Drawing for the job (mm, zero at the part's lowest x, y, z). A direction names the side the tool comes from. Coordinates: 2 decimals unless noted, no trailing zeros. Write each loop counter-clockwise with the first axis right and the second up, starting at its lowest first coordinate (ties: lowest second). Pieces come first, ordered by that corner, then holes. Notation, with made-up numbers: (33, 78.5) -> (71, 78.5) arc R29 ccw to (71, 105.5) -> close; hole circle Ø1 at (-29.5, 68). An arc over 180 degrees is marked (long way). Answer as CSV lines item,"result".
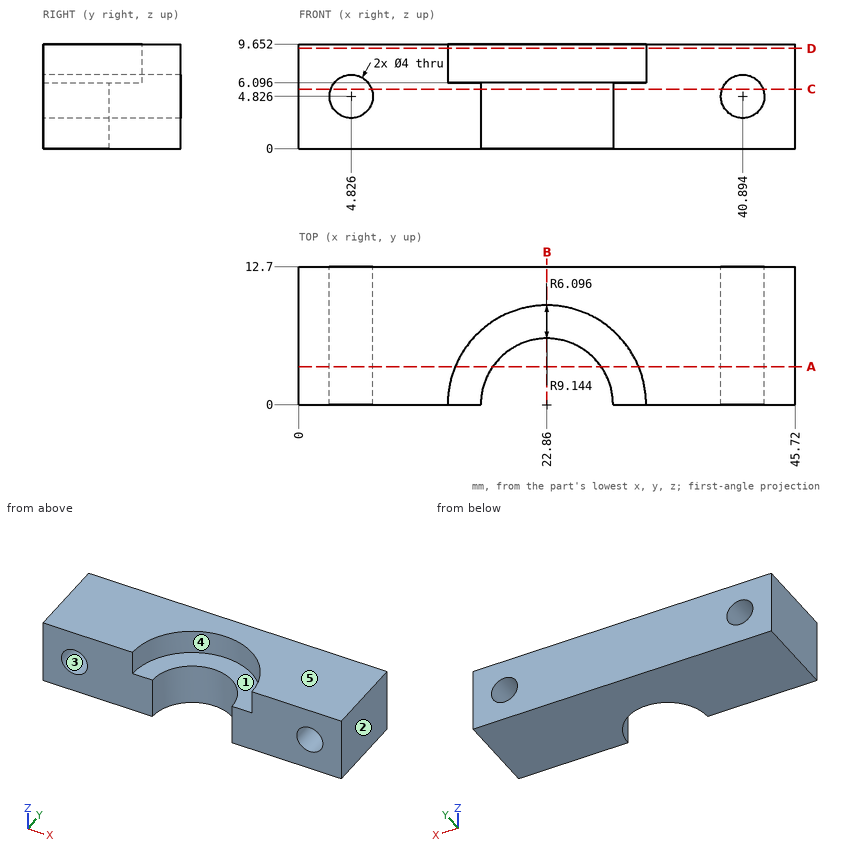
Item 1: Two-plate mould, pull along Z, no slides. Class the marked faces 3, 4 and 5: pulls with the +Z half, pulls with the -Z half, needs draft (parallel to the pull), parting line crosses it, or undercut.
Answer below:
face 3,"undercut"
face 4,"needs draft"
face 5,"pulls with the +Z half"
Item 2: 3-axis set-ups, long thin cutter, end or side, ignore diameter. For the marked faces 1 and 2: which of +Z, -Z, +X, -X, +Y, -Y reach the whole face in a straight line?
Answer below:
face 1,"+Z, -Y"
face 2,"+Z, -Z, +X, +Y, -Y"
Item 3: Wall check: line 1 (X direction, y = 8.5, z = 5); line 2 (X direction, y = 5.5, z = 6.5); line 3 (X direction, y = 3.75, z = 4.5). Give the ranges that are in metal, low to high. Write a range as from..to.
Answer below:
line 1,"x = 0..2.83, 6.82..38.9, 42.89..45.72"
line 2,"x = 0..3.73, 5.92..15.56, 30.16..39.8, 41.99..45.72"
line 3,"x = 0..2.85, 6.8..18.05, 27.67..38.92, 42.87..45.72"
Item 4: Flat gauge pin, fed straight in: pin 1 (6 mm diameter, centred on x = 26.5, y = 4.5, fed in from +Z). Where does the tip first touch, or does it go through?
Answer below:
pin 1,"stops at z = 6.1"
Item 5: Saw through at A-A on y = 3.5. Give the cut face in (x, z).
Answer below:
outline,"(0, 0) -> (17.87, 0) -> (17.87, 6.1) -> (14.41, 6.1) -> (14.41, 9.65) -> (0, 9.65) -> close; (27.85, 0) -> (45.72, 0) -> (45.72, 9.65) -> (31.31, 9.65) -> (31.31, 6.1) -> (27.85, 6.1) -> close; hole circle Ø4 at (4.83, 4.83); hole circle Ø4 at (40.89, 4.83)"
Item 6: Saw through at B-B on x = 22.86. Give the cut face in (y, z), and give its area (3 significant figures).
Answer below:
outline,"(6.1, 0) -> (12.7, 0) -> (12.7, 9.65) -> (9.14, 9.65) -> (9.14, 6.1) -> (6.1, 6.1) -> close"
area,"52.9 mm2"
Item 7: Saw through at D-D on z = 9.25. Give the cut face in (x, y).
Answer below:
outline,"(0, 0) -> (13.72, 0) arc R9.14 cw to (32, 0) -> (45.72, 0) -> (45.72, 12.7) -> (0, 12.7) -> close"
Item 8: Saw through at C-C on z = 5.5. Give the cut face in (x, y), and give its area (3 significant figures).
Answer below:
outline,"(0, 0) -> (2.94, 0) -> (2.94, 12.7) -> (0, 12.7) -> close; (6.71, 0) -> (16.76, 0) arc R6.1 cw to (28.96, 0) -> (39.01, 0) -> (39.01, 12.7) -> (6.71, 12.7) -> close; (42.78, 0) -> (45.72, 0) -> (45.72, 12.7) -> (42.78, 12.7) -> close"
area,"427 mm2"
